Geometry check sheet. Reference: the model listing, model coordinates, mm. Face numbers are marked on the shaded views. Coordinates: 2 decimals unless noted, no trailing zeros. Write each loop counter-clockwise with the first axis right and the second up, starting at its lowest first coordinate (ties: lowest second). Pieces come first, ordered by that corner, then holes. Notation, with made-up numbers: M -16.5,72 L 31.5,72 A14 ccw 31.5,92 Z; hole C 89.25,36.25 d8. An arc over 180 degrees is marked long. Write each question's results on one line, items separated by ' | '.
```python
from build123d import *

# Parameters (mm, degrees)
F0_R     = 40.456666
F0_R_2   = 22.253777
F1_DEPTH = 127
F2_DEPTH = 50
F3_R     = 5
F4_R     = 5


with BuildPart() as f1:
    # F0 (on Front) → F1 (new body)
    with BuildSketch(Plane.XZ):
        with Locations((-0.708535, -0.357763)):
            Circle(F0_R)
        Circle(F0_R_2, mode=Mode.SUBTRACT)
    extrude(amount=F1_DEPTH)

    # F0 (on Front) → F2 (join)
    with BuildSketch(Plane.XZ):
        with Locations((-0.708535, -0.357763)):
            Circle(F0_R)
        Circle(F0_R_2, mode=Mode.SUBTRACT)
    extrude(amount=F2_DEPTH)

    # F3
    f3_edges = [f1.edges().sort_by_distance(p)[0] for p in [
        (-41.165201, -127, -0.357763),
    ]]
    fillet(f3_edges, radius=F3_R)

    # F4
    f4_edges = [f1.edges().sort_by_distance(p)[0] for p in [
        (-22.253777, -127, 0),
    ]]
    fillet(f4_edges, radius=F4_R)


solid = f1.part
```
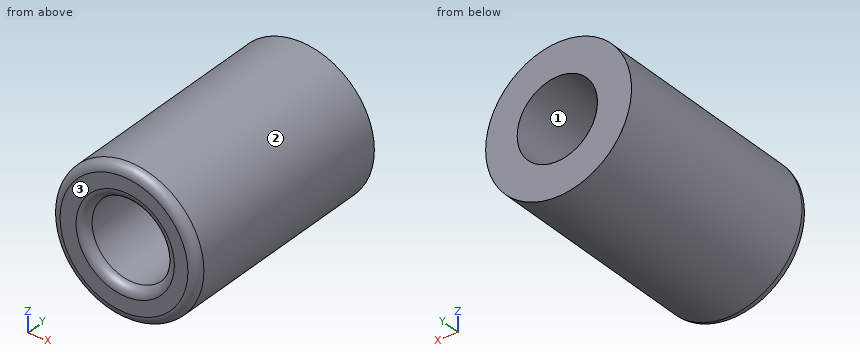
Q1. Depth check by flat-ended pin: P1, Ø3, axis at y = -46, z = 10, coming from the -X side; P2, Ø1.5, axis at y = -86, z = 12.5, coming from the -X side; P3, Ø2, axis at y = -107.5, z = 13, coming from the -X side; P4, Ø2, axis at x = 20.5, z = 1, coming from the -Y side. Enter the tip coordinate at first touch or a pass-through.
Geometry check:
P1: stops at x = -40.18 | P2: stops at x = -39.31 | P3: stops at x = -39.23 | P4: passes through
Q2. Sectioned sample at A-A on y = -74. Record the cut outline in (x, z).
Geometry check:
outline: C -0.71,-0.36 d80.91; hole C 0,0 d44.51
Q3. Scan lines: probe 1 along Z at (x, y) = (0, -90); probe 2 along Z at (x, y) = (-12, -32); probe 3 along X at (y, z) = (-107.5, -12). Record each from-to range of solid material in increasing order.
Geometry check:
probe 1: z = -40.81 to -22.25, 22.25 to 40.09 | probe 2: z = -39.21 to -18.74, 18.74 to 38.49 | probe 3: x = -39.45 to -18.74, 18.74 to 38.04
Q4. Mould release check, pull along X, two halves, no side actions. Record for the marked faces 1, 2 and 3: pulls with the +X half, pulls with the -X half, needs draft (parallel to the pull), parting line crosses it, or undercut.
Geometry check:
face 1: undercut | face 2: parting line crosses it | face 3: needs draft
